Work out the finished part from the listing and answer in its coordinate system (mm). Face numbers are marked on the shaded views. A direction names the side the tool comes from. Give positions to 0.01 mm unless a question says otherwise; leave off trailing zeros. Loops run counter-clockwise (first coordinate to the right, second up) from the corner with the lowest first, then second, coordinate; pieces in that order, holes last.
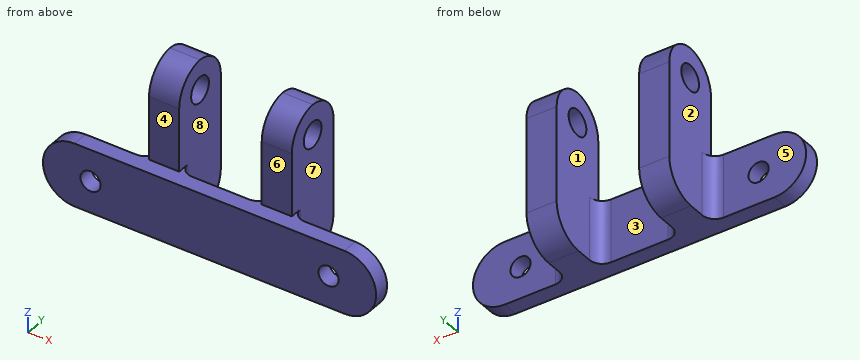
```python
from build123d import *

# Parameters (mm, degrees)
SKETCH1_W                   = 45
SKETCH1_H                   = 20
BOSS_EXTRUDE1_DEPTH         = 5
SKETCH2_W                   = 9.5
SKETCH2_H                   = 20
BOSS_EXTRUDE2_DEPTH         = 19.05
SKETCH3_W                   = 9.5
SKETCH3_H                   = 19.05
BOSS_EXTRUDE3_DEPTH         = 30
SKETCH4_R                   = 4.064
CUT_EXTRUDE1_DEPTH          = 65.833652527
SKETCH8_W                   = 30
SKETCH8_H                   = 20
BOSS_EXTRUDE4_DEPTH         = 5
F_1_4_0_25_DIAMETER_HOLE1_D = 6.35
FILLET1_R                   = 10
FILLET2_R                   = 4


with BuildPart() as part:
    # Sketch1 → Boss-Extrude1 (new body)
    with BuildSketch(Plane(origin=(0, 0, 0), x_dir=(1, 0, 0), z_dir=(0, 1, 0))):
        Rectangle(SKETCH1_W, SKETCH1_H)
    extrude(amount=BOSS_EXTRUDE1_DEPTH)

    # Sketch2 → Boss-Extrude2 (add)
    with BuildSketch(Plane(origin=(0, 5, 0), x_dir=(1, 0, 0), z_dir=(0, 1, 0))):
        with Locations((17.75, 0)):
            Rectangle(SKETCH2_W, SKETCH2_H)
        with Locations((-17.75, 0)):
            Rectangle(SKETCH2_W, SKETCH2_H)
    extrude(amount=BOSS_EXTRUDE2_DEPTH)

    # Sketch3 → Boss-Extrude3 (add)
    with BuildSketch(Plane.XY.offset(10)):
        with Locations((-17.75, 14.525)):
            Rectangle(SKETCH3_W, SKETCH3_H)
        with Locations((17.75, 14.525)):
            Rectangle(SKETCH3_W, SKETCH3_H)
    extrude(amount=BOSS_EXTRUDE3_DEPTH)

    # Sketch4 → Cut-Extrude1 (cut, through all)
    with BuildSketch(Plane(origin=(22.5, 0, 0), x_dir=(0, 0, -1), z_dir=(1, 0, 0))):
        with Locations((-30.475, 14.525)):
            Circle(SKETCH4_R)
    extrude(amount=-CUT_EXTRUDE1_DEPTH, mode=Mode.SUBTRACT)

    # Sketch8 → Boss-Extrude4 (add)
    with BuildSketch(Plane(origin=(0, 5, 0), x_dir=(1, 0, 0), z_dir=(0, 1, 0))):
        with Locations((37.5, 0)):
            Rectangle(SKETCH8_W, SKETCH8_H)
        with Locations((-37.5, 0)):
            Rectangle(SKETCH8_W, SKETCH8_H)
    extrude(amount=-BOSS_EXTRUDE4_DEPTH)

    # 1/4 (0.25) Diameter Hole1 (through all)
    with Locations(Plane(origin=(0, 5, 0), x_dir=(1, 0, 0), z_dir=(0, 1, 0))):
        with Locations((37.5, 0), (-37.5, 0)):
            Hole(F_1_4_0_25_DIAMETER_HOLE1_D / 2)

    # Fillet1
    # the kernel refuses this fillet: 10 mm, written as the material it takes off along each edge
    with BuildSketch(Plane(origin=(-47.5, 24.05, -10), x_dir=(0, -1, 0), z_dir=(1, 0, 0)), Plane(origin=(12, 5, 40), x_dir=(0, 0, -1), z_dir=(-1, 0, 0)), Plane(origin=(47.5, 5, 40), x_dir=(0, 0, -1), z_dir=(-1, 0, 0))) as fillet1_piece_1:
        with BuildLine():
            CenterArc((FILLET1_R, -FILLET1_R), FILLET1_R, 90, 90)
            Line((0, -FILLET1_R), (0, 0))
            Line((0, 0), (FILLET1_R, 0))
        make_face()
    extrude(amount=59.5, mode=Mode.SUBTRACT)
    with BuildSketch(Plane(origin=(-47.5, 24.05, 40), x_dir=(0, -1, 0), z_dir=(1, 0, 0)), Plane(origin=(-12, 24.05, 40), x_dir=(0, -1, 0), z_dir=(1, 0, 0)), Plane(origin=(47.5, 24.05, -10), x_dir=(0, -1, 0), z_dir=(-1, 0, 0))) as fillet1_piece_2:
        with BuildLine():
            CenterArc((FILLET1_R, FILLET1_R), FILLET1_R, 180, 90)
            Line((0, FILLET1_R), (0, 0))
            Line((0, 0), (FILLET1_R, 0))
        make_face()
    extrude(amount=59.5, mode=Mode.SUBTRACT)
    with BuildSketch(Plane(origin=(52.5, 30, 10), x_dir=(-1, 0, 0), z_dir=(0, -1, 0)), Plane(origin=(52.5, 30, -10), x_dir=(0, 0, 1), z_dir=(0, -1, 0))) as fillet1_piece_3:
        with BuildLine():
            CenterArc((FILLET1_R, FILLET1_R), FILLET1_R, 180, 90)
            Line((0, FILLET1_R), (0, 0))
            Line((0, 0), (FILLET1_R, 0))
        make_face()
    extrude(amount=55, mode=Mode.SUBTRACT)
    with BuildSketch(Plane(origin=(-52.5, 30, 10), x_dir=(1, 0, 0), z_dir=(0, -1, 0)), Plane(origin=(-52.5, 30, -10), x_dir=(0, 0, 1), z_dir=(0, -1, 0))) as fillet1_piece_4:
        with BuildLine():
            CenterArc((FILLET1_R, -FILLET1_R), FILLET1_R, 90, 90)
            Line((0, -FILLET1_R), (0, 0))
            Line((0, 0), (FILLET1_R, 0))
        make_face()
    extrude(amount=55, mode=Mode.SUBTRACT)

    # Fillet2
    fillet2_edges = [part.edges().sort_by_distance(p)[0] for p in [
        (13, 5, 0),
        (-13, 5, 0),
        (22.5, 5, 0),
        (-22.5, 5, 0),
    ]]
    fillet(fillet2_edges, radius=FILLET2_R)


solid = part.part
```
Q1. Given pin 1 (10 mm diameter, centred on x = -20, y = 5, fed in from +Z); pin 2 (5.5 mm diameter, centred on y = 16, z = 13, fed in from -X); pin 3 (3 mm diameter, centred on x = 19.5, z = 19, fed in from -Y); pin 4 (5 mm diameter, centred on y = 14.525, z = 30.475, fed in from -X), each flat-ended and moving along its own axis, determine where each tip first touches the part or whether it passes through.
Q2. Determine the mould class of the marked faces 6, 7 and 8 for opening direction X: +X half, -X half, draft (parallel to the pull), parting line (faces both ways), or undercut.
Q3. Section C-C on x = 19.5 is taken. Give the vertices of the cut face in (y, z) (3 decimals).
Q4. Section A-A on x = 37.5 is taken. Give the vertices of the cut face in (y, z) (3 decimals), plus the area to 4 significant figures.
Q5. Section D-D on x = -29 is taken. Give the vertices of the cut face in (y, z), plus the area to 3 significant figures.
Q6. Consider line 1 along X through (y, z) = (6.25, 19.5); line 2 along Y through (x, z) = (20, -0.5); line 3 along Z through (x, y) = (-37.5, 1.1) (3 decimals). Determine where each line is inside the solid, lowest interval first.
Q7. Which of the six approach directions +Z, -Z, +X, -X, +Y, -Y give full straight-line access (tool end or side, diameter ignored) to the marked faces 1, 2, 3, 4 and 5?
Q8. Section B-B on z = -6 is taken. Give the vertices of the cut face in (x, y).
Check result:
1. pin 1: stops at z = 38.66
1. pin 2: stops at x = -22.5
1. pin 3: stops at y = 5
1. pin 4: passes through
2. face 6: draft
2. face 7: +X half
2. face 8: undercut
3. outline: (0, -10) - (14.05, -10) arc R10 ccw to (24.05, 0) - (24.05, 30) arc R10 ccw to (14.525, 39.989) arc R10 ccw to (5, 30) - (5, 10) - (0, 10) - close; hole circle Ø8.128 at (14.525, 30.475)
4. outline: (0, -10) - (5, -10) - (5, -3.175) - (0, -3.175) - close; (0, 3.175) - (5, 3.175) - (5, 10) - (0, 10) - close
4. area: 68.25 mm2
5. outline: (0, -10) - (5, -10) - (5, 10) - (0, 10) - close
5. area: 100 mm2
6. line 1: x = -22.5 to -13, 13 to 22.5
6. line 2: y = 0 to 24.04
6. line 3: z = -10 to -3.175, 3.175 to 10
7. face 1: +Z, +Y
7. face 2: +Z, -X, +Y
7. face 3: +Z, -Z, +Y
7. face 4: +Z, +X, -X, -Y
7. face 5: +Z, -Z, -X, +Y
8. outline: (-50.5, 0) - (50.5, 0) - (50.5, 5) - (26.5, 5) arc R4 cw to (22.5, 9) - (22.5, 22.05) - (13, 22.05) - (13, 9) arc R4 cw to (9, 5) - (-9, 5) arc R4 cw to (-13, 9) - (-13, 22.05) - (-22.5, 22.05) - (-22.5, 9) arc R4 cw to (-26.5, 5) - (-50.5, 5) - close
